from build123d import *

# Parameters (mm, degrees)
SKETCH1_R                       = 82.55
BOSS_EXTRUDE1_DEPTH             = 3.81
HOLE1_OUTLINE_R                 = 12.7
HOLE1_DEPTH                     = 3.81
BOSS_EXTRUDE2_START             = 0.0254
SKETCH3_R                       = 82.55
SKETCH3_R_2                     = 78.74
BOSS_EXTRUDE2_DEPTH             = 0.0254
SKETCH4_R                       = 6
BOSS_EXTRUDE3_DEPTH             = 1.27
SKETCH5_R                       = 3.75
BOSS_EXTRUDE4_DEPTH             = 6
SKETCH7_W                       = 42
SKETCH7_H                       = 42
BOSS_EXTRUDE5_DEPTH             = 3
SKETCH8_R                       = 11.25
CUT_EXTRUDE2_DEPTH              = 2.5
CUT_EXTRUDE1_DEPTH              = 118.267947027
CUT_EXTRUDE1_DEPTH_BACK         = 118.267947027
SKETCH6_R                       = 3
CBORE_FOR_M3_SBHCS1_D           = 3.4
CBORE_FOR_M3_SBHCS1_CBORE_D     = 6.7
CBORE_FOR_M3_SBHCS1_CBORE_DEPTH = 1.65
SKETCH12_W                      = 6.604
SKETCH12_H                      = 13.462
CUT_EXTRUDE3_DEPTH              = 1.27
SKETCH13_W                      = 2.794
SKETCH13_H                      = 2.794
CUT_EXTRUDE4_DEPTH              = 2.794
CUT_EXTRUDE5_DEPTH              = 118.05527156


# Read off the part's stored shape, not the designer's step: Hole1, Lip1
with BuildPart() as part:
    # Sketch1 → Boss-Extrude1 (new body)
    with BuildSketch(Plane(origin=(0, 0, 0), x_dir=(1, 0, 0), z_dir=(0, 1, 0))):
        with Locations(Location((0, 0, 0), (0, 0, 90))):
            Circle(SKETCH1_R)
    extrude(amount=BOSS_EXTRUDE1_DEPTH)

    # Hole1 outline → Hole1 (cut)
    with BuildSketch(Plane(origin=(0, 0, 0), x_dir=(1, 0, 0), z_dir=(0, 1, 0))):
        with Locations((-0.958051057, 57.141969149)):
            Circle(HOLE1_OUTLINE_R)
    extrude(amount=HOLE1_DEPTH, mode=Mode.SUBTRACT)

    # Sketch3 → Boss-Extrude2 (add)
    with BuildSketch(Plane.XZ.offset(BOSS_EXTRUDE2_START)):
        with Locations(Location((0, 0, 0), (0, 0, 270))):
            Circle(SKETCH3_R)
        with Locations(Location((0, 0, 0), (0, 0, 270))):
            Circle(SKETCH3_R_2, mode=Mode.SUBTRACT)
    extrude(amount=-BOSS_EXTRUDE2_DEPTH)

    # Lip1 outline → Lip1 (revolve)
    with BuildSketch(Plane.XY):
        Polygon((78.74, -0.0254), (78.74, -1.8034), (80.424818968, -1.8034), (80.518, -0.0254), align=None)
    revolve(axis=Axis((0, 0, 0), (0, 1, 0)))

    # Sketch4 → Boss-Extrude3 (add)
    with BuildSketch(Plane.XZ):
        with Locations(Location((0, 0, 0), (0, 0, 90))):
            Circle(SKETCH4_R)
    extrude(amount=BOSS_EXTRUDE3_DEPTH)

    # Sketch5 → Boss-Extrude4 (add)
    with BuildSketch(Plane.XZ.offset(1.27)):
        with Locations(Location((0, 0, 0), (0, 0, 270))):
            Circle(SKETCH5_R)
    extrude(amount=BOSS_EXTRUDE4_DEPTH)

    # Sketch7 → Boss-Extrude5 (add)
    with BuildSketch(Plane(origin=(0, 3.81, 0), x_dir=(1, 0, 0), z_dir=(0, 1, 0))):
        Rectangle(SKETCH7_W, SKETCH7_H)
    extrude(amount=BOSS_EXTRUDE5_DEPTH)

    # Sketch8 → Cut-Extrude2 (cut)
    with BuildSketch(Plane(origin=(0, 6.81, 0), x_dir=(1, 0, 0), z_dir=(0, 1, 0))):
        with Locations(Location((0, 0, 0), (0, 0, 270))):
            Circle(SKETCH8_R)
    extrude(amount=-CUT_EXTRUDE2_DEPTH, mode=Mode.SUBTRACT)

    # Sketch6 → Cut-Extrude1 (cut, two sides: drawn at the far end of the back side and taken through both)
    with BuildSketch(Plane(origin=(0, 3.81, 0), x_dir=(1, 0, 0), z_dir=(0, 1, 0)).offset(-CUT_EXTRUDE1_DEPTH_BACK)):
        with Locations(Location((0, 0, 0), (0, 0, 270))):
            Circle(SKETCH6_R)
    extrude(amount=CUT_EXTRUDE1_DEPTH + CUT_EXTRUDE1_DEPTH_BACK, mode=Mode.SUBTRACT)

    # CBORE for M3 SBHCS1 (through all)
    with Locations(Plane(origin=(0, 0, 0), x_dir=(-1, 0, 0), z_dir=(0, -1, 0))):
        with Locations((-15.5, 15.5), (-15.5, -15.5), (15.5, -15.5), (15.5, 15.5)):
            CounterBoreHole(CBORE_FOR_M3_SBHCS1_D / 2, CBORE_FOR_M3_SBHCS1_CBORE_D / 2, CBORE_FOR_M3_SBHCS1_CBORE_DEPTH)

    # Sketch12 → Cut-Extrude3 (cut)
    with BuildSketch(Plane.XZ):
        with Locations((-0.114811482, -27.731)):
            Rectangle(SKETCH12_W, SKETCH12_H)
        Polygon((13.368272935, -41.371347413), (19.479984235, -38.869387984), (14.379836168, -26.410899564), (8.268124867, -28.912858993), align=None)
    extrude(amount=-CUT_EXTRUDE3_DEPTH, mode=Mode.SUBTRACT)

    # Sketch13 → Cut-Extrude4 (cut)
    with BuildSketch(Plane.XZ.offset(-1.27)):
        with Locations((-0.114811482, -27.731)):
            Rectangle(SKETCH13_W, SKETCH13_H)
        Polygon((13.110453194, -35.713246143), (12.051931897, -33.127522131), (14.637655908, -32.069000834), (15.696177205, -34.654724846), align=None)
    extrude(amount=-CUT_EXTRUDE4_DEPTH, mode=Mode.SUBTRACT)

    # Sketch14 → Cut-Extrude5 (cut, through all)
    with BuildSketch(Plane.XZ.offset(-1.27)):
        with BuildLine():
            Line((1.155188518, -33.8905), (-1.384811482, -33.8905))
            ThreePointArc((-1.384811482, -33.8905), (-2.654811482, -32.6205), (-1.384811482, -31.3505))
            Line((-1.384811482, -31.3505), (1.155188518, -31.3505))
            ThreePointArc((1.155188518, -31.3505), (2.425188518, -32.6205), (1.155188518, -33.8905))
        make_face()
        with BuildLine():
            Line((-1.392065738, -21.683846113), (1.147892825, -21.669337601))
            ThreePointArc((1.147892825, -21.669337601), (2.425126363, -22.932062627), (1.162401338, -24.209296164))
            Line((1.162401338, -24.209296164), (-1.377557226, -24.223804677))
            ThreePointArc((-1.377557226, -24.223804677), (-2.654790763, -22.961079651), (-1.392065738, -21.683846113))
        make_face()
        with BuildLine():
            Line((10.365167141, -28.671923416), (12.715825333, -27.709631328))
            ThreePointArc((12.715825333, -27.709631328), (14.372300474, -28.40381438), (13.678117422, -30.06028952))
            Line((13.678117422, -30.06028952), (11.327459229, -31.022581609))
            ThreePointArc((11.327459229, -31.022581609), (9.670984089, -30.328398556), (10.365167141, -28.671923416))
        make_face()
        with BuildLine():
            Line((15.032283769, -40.072615649), (17.382941961, -39.110323561))
            ThreePointArc((17.382941961, -39.110323561), (18.077125013, -37.453848421), (16.420649873, -36.759665368))
            Line((16.420649873, -36.759665368), (14.069991681, -37.721957457))
            ThreePointArc((14.069991681, -37.721957457), (13.375808628, -39.378432597), (15.032283769, -40.072615649))
        make_face()
    extrude(amount=-CUT_EXTRUDE5_DEPTH, mode=Mode.SUBTRACT)


solid = part.part
CAD build for the part. Positions are in the model's coordinates, mm. A direction names the side the tool comes from. Round coordinates to 2 decimals unless told otherwise and drop trailing zeros. Order: outer loops, then holes, each group sorted by start corner. A loop starts at its lowest first (then second) coordinate and runs counter-clockwise, first axis right, second up. Notation, with made-up numbers: M 68.25,-37.75 L 113.25,-37.75 A23 cw 113.25,-13.75 Z; hole C 23.5,-35 d7. An arc over 180 degrees is marked long. Use one line per item in the form item = value.
Q1. Two-plate mould, pull along X, no slides. Class faces 1 (the flat face through (14, 1.65, 17)), 2 (the flat face through (-79, -0.025, -18)), 3 (the cylindrical face through (81.848, 1.865, 10.746)): +X half, -X half, draft (parallel to the pull), parting line (faces both ways), or undercut.
Recorded:
face_1 = undercut
face_2 = draft
face_3 = parting line
Q2. Which spindle directions (+Z, -Z, +X, -X, +Y, -Y) get a long thin tool onto all of the face, cutting with end or side? Do faces 4 (the cylindrical face through (-3.711, 1.878, -44.744)), 5 (the flat face through (3, -1.27, -3)), 6 (the flat face through (-2.3, 4.31, 2.3)). Say none if no direction does.
Recorded:
face_4 = +Y, -Y
face_5 = -Y
face_6 = +Y
Q3. Saw through at A-A on y = -4.5. Give the cut face in (x, z).
Recorded:
outline = C 0,0 d7.5; hole C 0,0 d6
Q4. Flat gauge pins, fed straight in: P1, Ø2, axis at x = 26.5, y = -0.5, coming from the -Z side; P2, Ø7, axis at x = 0, z = 5, coming from the +Y side; P3, Ø3, axis at x = -41, z = 21, coming from the -Y side. Where does each tip first touch, or does it go through?
Recorded:
P1 = -78.47
P2 = 4.31
P3 = 0
Q5. Probe L1, parallel to Z at x = -15.5, y = 5.75; L2, parallel to X at y = 0.4, z = 15.5; L3, parallel to Y at x = -65, z = -33.5. List the from-to ranges inside material, lowest first.
Recorded:
L1 = -21 to -17.2, -13.8 to 13.8, 17.2 to 21
L2 = -81.08 to -18.85, -12.15 to 12.15, 18.85 to 81.08
L3 = 0 to 3.81
